Could you check a few things on this model? Use its own coordinates, in mm. A direction names the side the tool comes from. Round coordinates to 2 decimals unless told otherwise and drop trailing zeros. Loops run counter-clockwise (first coordinate to the right, second up) from the corner with the lowest first, then second, coordinate; pieces in that order, holes last. Notation, with made-up numbers: M 56.25,25.5 L 63.25,25.5 A12 ccw 63.25,29.5 Z; hole C -38,27.5 d6. An arc over 180 degrees is marked long. One line per item, written item: value. Start each with the question number.
Q1. Please list where these lines run through material, in increasing order: line 1 along X through (y, z) = (265, -215.5); line 2 along Y through (x, z) = (-3.5, -493); line 3 along Z through (x, y) = (-1.25, 240).
Q2. Thinking about a two-plate mould opening in Y: for faces 1 (the face through (-4.4, 145, -112)), 2 (the face through (-2.2, 207.4, -170.9)), 3 (the face through (-2.17, 257.18, -258.88)), 4 (the face through (-2.17, 285.96, -516.13)), which applies, released by +Y, released by -Y, zero draft, split by the parting line, or undercut?
Q3. Imagine slicing it at A-A (z = -92). Please give me the cut outline in (x, y), then the cut area to 3 significant figures.
Q4. Imagine slicing it at B-B (x = -2.5). Please give me the cut outline in (y, z).
Q5. Imagine slicing it at D-D (y = 19). Please give me the cut outline in (x, z).
Q6. Imagine slicing it at C-C (z = -163). Please give me the cut outline in (x, y), then the cut area to 3 significant figures.
Q7. Which directions (+Z, -Z, +X, -X, +Y, -Y) give clear straight access to the entire face, cutting with the end or side of a thin tool? Please do faces 5 (the face through (-2.17, 130.92, -108.05)), 6 (the face through (-2.17, 278.03, -253.44)), 7 (the face through (-2.2, 266.2, -512.5)).
Q8. I'm going to push a flat-ended pin straight in: pin 1 Ø3.5 at (x, z) = (-1.5, -372) entering from -Y. Where does the tip first touch, or does it pass through?
from build123d import *

# Parameters (mm, degrees)
BOSS_EXTRUDE1_DEPTH = 4.4
BOSS_EXTRUDE2_DEPTH = 4.4


with BuildPart() as part:
    # Sketch1 → Boss-Extrude1 (new body)
    with BuildSketch(Plane(origin=(0, 0, 0), x_dir=(0, 0, -1), z_dir=(1, 0, 0))):
        with BuildLine():
            Line((12.615293263, -92.633282396), (182.615293263, -92.633282396))
            ThreePointArc((182.615293263, -92.633282396), (98.271459614, -21.762843967), (84.825943994, 87.579368501))
            Line((84.825943994, 87.579368501), (131.929787104, 175.483372313))
            Line((131.929787104, 175.483372313), (210.884858569, 240.150484061))
            Line((210.884858569, 240.150484061), (308.236471933, 274.689971372))
            Line((308.236471933, 274.689971372), (415.1194685, 274.721469403))
            Line((415.1194685, 274.721469403), (612.615293263, 257.442823643))
            ThreePointArc((612.615293263, 257.442823643), (623.448797672, 266.533213196), (614.358408118, 277.366717604))
            Line((614.358408118, 277.366717604), (415.1194685, 294.797866154))
            Line((415.1194685, 294.797866154), (305.051694272, 294.797866154))
            Line((305.051694272, 294.797866154), (200.371020359, 260.785053385))
            Line((200.371020359, 260.785053385), (111.324320476, 196.088838941))
            Line((111.324320476, 196.088838941), (46.628106033, 107.042139058))
            Line((46.628106033, 107.042139058), (12.615293263, 2.361465145))
            Line((12.615293263, 2.361465145), (12.615293263, -92.633282396))
        make_face()
    extrude(amount=-BOSS_EXTRUDE1_DEPTH)

    # Sketch2 → Boss-Extrude2 (add)
    with BuildSketch(Plane.ZY.offset(4.4)):
        with BuildLine():
            Line((-614.358408118, 277.366717604), (-614.079509741, 274.178894571))
            Line((-614.079509741, 274.178894571), (-609.098536251, 274.614673284))
            Line((-609.098536251, 274.614673284), (-607.91321815, 261.06642539))
            Line((-607.91321815, 261.06642539), (-612.89419164, 260.630646676))
            Line((-612.89419164, 260.630646676), (-612.615293263, 257.442823643))
            ThreePointArc((-612.615293263, 257.442823643), (-623.448797672, 266.533213196), (-614.358408118, 277.366717604))
        make_face()
    extrude(amount=BOSS_EXTRUDE2_DEPTH)


solid = part.part
Report:
1. line 1: x = -4.4 to 0
1. line 2: y = 267.91 to 287.98
1. line 3: z = -210.7 to -171.76
2. face 1: zero draft
2. face 2: undercut
2. face 3: released by -Y
2. face 4: released by +Y
3. outline: M -4.4,-92.63 L 0,-92.63 L 0,-8.75 L -4.4,-8.75 Z; M -4.4,100.97 L 0,100.97 L 0,169.49 L -4.4,169.49 Z
3. area: 671 mm²
4. outline: M -92.63,-182.62 A150.46 cw 87.58,-84.83 L 175.48,-131.93 L 240.15,-210.88 L 274.69,-308.24 L 274.72,-415.12 L 257.44,-612.62 A10 ccw 277.37,-614.36 L 294.8,-415.12 L 294.8,-305.05 L 260.79,-200.37 L 196.09,-111.32 L 107.04,-46.63 L 2.36,-12.62 L -92.63,-12.62 Z
5. outline: M -4.4,-83.28 L 0,-83.28 L 0,-18.02 L -4.4,-18.02 Z
6. outline: M -4.4,-92.63 L 0,-92.63 L 0,-84.46 L -4.4,-84.46 Z; M -4.4,200.93 L 0,200.93 L 0,233.63 L -4.4,233.63 Z
6. area: 180 mm²
7. face 5: -Z, +X, -X
7. face 6: +Z, +X, -X, +Y
7. face 7: +X, -X, -Y
8. pin 1: stops at y = 274.71
